Input: part model. Units: mm. Frame: model coordinates. A direction names the side the tool comes from. Coordinates: 2 decimals unless noted, no trailing zeros. Write each loop counter-clockwise with the first axis right and the second up, starting at its lowest first coordinate (ties: lowest second). Pieces come first, ordered by that corner, then holes.
1) Section query C-C (z = -16.5). Output: boundary loops of the cut face in (x, y), then the cut area to 3 significant figures.
2) Line query: L1, parallel to X at y = 18, z = -8.5; L2, parallel to Y at x = -9, z = -1.5; L3, parallel to Z at x = -17.75, y = -20 (3 decimals). Output: solid intervals per line, ascending.
3) Pin query (flat end, axial travel): pin 1 Ø1.4 at (x, y) = (2, -4) entering from -Z; pin 2 Ø9.5 at (x, y) = (-13, 16) entering from -Z (3 decimals); pin 3 Ø2 at (y, z) = (-6, -4.5) entering from -X; pin 4 Ø12 at (x, z) = (-4, -15) entering from -Y. Return the tip coordinate at first contact, or that it passes through.
4) Section query A-A (x = -13.75). Output: boundary loops of the cut face in (y, z) (3 decimals).
5) Set-up query: faces 1 (the flat face through (-0.79, -11.86, 2.55)), 2 (the cylindrical face through (2.35, 26.93, -31.75)), 3 (the flat face through (-10, -12.7, -1)), 4 (the flat face through (2, -22.225, -26)), 5 (the flat face through (-6.023, -31.106, 2.549)). Return all of +Z, -Z, +X, -X, +Y, -Y with unobstructed straight access to the full face (end or side cutting, diameter ignored); none if empty.
6) Section query B-B (x = 2). State how many separate pieces and enclosed holes the cut face has, then the cut area to 3 significant figures.
7) Draft query along Z for faces 6 (the flat face through (2, 0, -7.938)), 7 (the flat face through (-17.31, 30.04, 2.55)), 8 (the flat face through (4.762, 0.4, -7.7)), 9 (the flat face through (2, -29.445, -25)). Return one class per face: pulls with the +Z half, pulls with the -Z half, needs draft (parallel to the pull), parting line crosses it, or undercut.
from build123d import *

# Parameters (mm, degrees)
SKETCH1_W                 = 6.35
SKETCH1_H                 = 63.5
BOSS_EXTRUDE1_DEPTH       = 19.05
BOSS_EXTRUDE2_DEPTH       = 4.7625
SKETCH4_W                 = 19.05
SKETCH4_H                 = 25.4
CUT_EXTRUDE1_DEPTH        = 6.35
CHAMFER1_SIZE             = 12.7
CHAMFER2_SIZE             = 2.54
CHAMFER3_SIZE             = 1.27
F_8_CLEARANCE_SLOT1_DEPTH = 4.7625


# Read off the part's stored shape, not the designer's step: #8 Clearance Slot1
with BuildPart() as part:
    # Sketch1 → Boss-Extrude1 (new body)
    with BuildSketch(Plane(origin=(0, 0, 0), x_dir=(0, 0, -1), z_dir=(1, 0, 0))):
        Rectangle(SKETCH1_W, SKETCH1_H)
    extrude(amount=-BOSS_EXTRUDE1_DEPTH)

    # Sketch2 → Boss-Extrude2 (add)
    with BuildSketch(Plane(origin=(0, 0, 0), x_dir=(0, 0, -1), z_dir=(1, 0, 0))):
        Polygon((-3.175, 31.75), (34.925, 31.75), (34.925, 22.225), (7.9375, 22.225), (7.9375, -22.225), (34.925, -22.225), (34.925, -31.75), (-3.175, -31.75), align=None)
    extrude(amount=BOSS_EXTRUDE2_DEPTH)

    # Sketch4 → Cut-Extrude1 (cut)
    with BuildSketch(Plane.XY.offset(3.175)):
        with Locations((-9.525, 0)):
            Rectangle(SKETCH4_W, SKETCH4_H)
    extrude(amount=-CUT_EXTRUDE1_DEPTH, mode=Mode.SUBTRACT)

    # Chamfer1
    chamfer1_edges = [part.edges().sort_by_distance(p)[0] for p in [
        (2.38125, -22.225, -7.9375),
        (2.38125, 22.225, -7.9375),
    ]]
    chamfer(chamfer1_edges, length=CHAMFER1_SIZE)

    # Chamfer2
    chamfer2_edges = [part.edges().sort_by_distance(p)[0] for p in [
        (-19.05, 31.75, 0),
        (2.38125, -31.75, -34.925),
        (2.38125, -22.225, -34.925),
        (2.38125, 22.225, -34.925),
        (2.38125, 31.75, -34.925),
        (-19.05, -12.7, 0),
        (-19.05, 12.7, 0),
        (0, 12.7, 0),
        (0, -12.7, 0),
        (-19.05, -31.75, 0),
    ]]
    chamfer(chamfer2_edges, length=CHAMFER2_SIZE)

    # Chamfer3
    chamfer3_edges = [part.edges().sort_by_distance(p)[0] for p in [
        (-9.525, 12.7, 3.175),
        (0, 0, 3.175),
        (-9.525, -12.7, 3.175),
        (-19.05, -22.225, 3.175),
        (-5.87375, -31.75, 3.175),
        (-5.87375, 31.75, 3.175),
        (-19.05, 22.225, 3.175),
        (-17.78, 30.48, 3.175),
        (-17.78, -30.48, 3.175),
        (-17.78, 13.97, 3.175),
        (-17.78, -13.97, 3.175),
        (-1.27, 11.43, 3.175),
        (-1.27, -11.43, 3.175),
    ]]
    chamfer(chamfer3_edges, length=CHAMFER3_SIZE)

    # #8 Clearance Slot1 outline → #8 Clearance Slot1 (cut)
    with BuildSketch(Plane.YZ):
        with BuildLine():
            Line((-24.53005, -29.29255), (-24.53005, -21.50745))
            ThreePointArc((-24.53005, -21.50745), (-26.9875, -19.05), (-29.44495, -21.50745))
            Line((-29.44495, -21.50745), (-29.44495, -29.29255))
            ThreePointArc((-29.44495, -29.29255), (-26.9875, -31.75), (-24.53005, -29.29255))
        make_face()
        with BuildLine():
            Line((24.53005, -21.50745), (24.53005, -29.29255))
            ThreePointArc((24.53005, -29.29255), (26.9875, -31.75), (29.44495, -29.29255))
            Line((29.44495, -29.29255), (29.44495, -21.50745))
            ThreePointArc((29.44495, -21.50745), (26.9875, -19.05), (24.53005, -21.50745))
        make_face()
    extrude(amount=F_8_CLEARANCE_SLOT1_DEPTH, mode=Mode.SUBTRACT)


solid = part.part
Answer:
1. outline: (0, -31.75) - (4.76, -31.75) - (4.76, -18.09) - (0, -18.09) - close; (0, 18.09) - (4.76, 18.09) - (4.76, 31.75) - (0, 31.75) - close
1. area: 130 mm2
2. L1: x = 0 to 4.76
2. L2: y = -31.75 to -12.7, 12.7 to 31.75
2. L3: z = -3.175 to 3.175
3. pin 1: stops at z = -7.94
3. pin 2: stops at z = -3.175
3. pin 3: stops at x = 0
3. pin 4: stops at y = -31.75
4. outline: (-31.75, -3.175) - (-12.7, -3.175) - (-12.7, 1.905) - (-13.97, 3.175) - (-30.48, 3.175) - (-31.75, 1.905) - close; (12.7, -3.175) - (31.75, -3.175) - (31.75, 1.905) - (30.48, 3.175) - (13.97, 3.175) - (12.7, 1.905) - close
5. face 1: +Z, -X
5. face 2: +X, -X
5. face 3: +Z, -Z, -X
5. face 4: -Z, +X, -X
5. face 5: +Z, +X, -X, -Y
6. separate pieces: 1
6. enclosed holes: 2
6. area: 1,250 mm2
7. face 6: pulls with the -Z half
7. face 7: pulls with the +Z half
7. face 8: needs draft
7. face 9: undercut
